Autodesk Inventor part; units mm, degrees
ref_plane "YZ Plane" through (0, 0, 0) normal (1, 0, 0) x (0, 1, 0)
ref_plane "XZ Plane" through (0, 0, 0) normal (0, 1, 0) x (-1, 0, 0)
ref_plane "XY Plane" through (0, 0, 0) normal (0, 0, 1) x (1, 0, 0)
sketch "Sketch1" plane through (0, 0, 0) normal (0, 0, 1) x (1, 0, 0)
  line L0 (-2.54, -8.19) -> (2.54, -8.19)
  line L1 (2.54, -8.19) -> (2.54, 8.19)
  line L2 (-2.54, 8.19) -> (-2.54, -8.19)
  line L3 (-2.54, -8.19) -> (2.54, 8.19) construction
  line L4 (2.54, -8.19) -> (-2.54, 8.19) construction
  circle A0 centre (0, 16.6545) radius 2.5 construction
  circle A1 centre (0, 16.6545) radius 5
  arc A2 (6.8029, 15.0051) -> (-6.8044, 15.0114) centre (0, 16.6545) ccw
  line L5 (-2.54, 8.19) -> (-2.54, 10.2591)
  line L6 (2.54, 8.19) -> (2.54, 10.2869)
  line L7 (0, 0) -> (0, 10.7842) construction
  line L8 (-2.54, 10.2591) -> (-3.9944, 10.2511)
  line L9 (2.54, 10.2869) -> (3.9944, 10.2948)
  line L10 (-3.9944, 10.2511) -> (-4.1214, 3.9003)
  line L11 (3.9944, 10.2948) -> (4.1214, 3.9454)
  line L12 (-4.1214, 3.9003) -> (-6.8044, 15.0114)
  line L13 (4.1214, 3.9454) -> (6.8029, 15.0051)
  line L14 (0, 0) -> (0, 22.9511) construction
  point P0 (-3.2672, 10.2551)
  dimension "d2" = 5
  dimension "d3" = 10
  dimension "d4" = 14
  dimension "d8" = 1.5815
  dimension "d9" = 1.5815
  dimension "d10" = 6.35
  dimension "d11" = 6.35
  dimension "d18" = 1.4545
  dimension "d19" = 1.4545
  dimension "d31" = 2.54
  dimension "d32" = 2.54
  dimension "d33" = 0
extrude "Plate1" add sketch "Sketch1" along normal blind 1.5748
sketch "Sketch2" plane through (0, 0, 0) normal (0, 0, -1) x (-1, 0, 0)
  circle A0 centre (0, 16.6545) radius 5
  line L0 (-3.9944, 10.2948) -> (-4.1214, 3.9454)
  line L1 (-2.54, 10.2869) -> (-3.9944, 10.2948)
  line L2 (-2.54, -8.19) -> (-2.54, 10.2869)
  line L3 (2.54, -8.19) -> (-2.54, -8.19)
  line L4 (2.54, 10.2591) -> (2.54, -8.19)
  line L5 (3.9944, 10.2511) -> (2.54, 10.2591)
  line L6 (4.1214, 3.9003) -> (3.9944, 10.2511)
  line L7 (6.8044, 15.0114) -> (4.1214, 3.9003)
  arc A1 (6.8044, 15.0114) -> (-6.8029, 15.0051) centre (0, 16.6545) ccw
  line L8 (-4.1214, 3.9454) -> (-6.8029, 15.0051)
  line L9 (-1.5875, -17.19) -> (1.5875, -17.19)
  line L10 (1.5875, -17.19) -> (1.5875, 0.81)
  line L11 (1.5875, 0.81) -> (-1.5875, 0.81)
  line L12 (-1.5875, 0.81) -> (-1.5875, -17.19)
  line L13 (-1.5875, -17.19) -> (1.5875, 0.81) construction
  line L14 (1.5875, -17.19) -> (-1.5875, 0.81) construction
  point P0 (0, 0)
  point P1 (0, -8.19)
  dimension "d14" = 3.175
extrude "Extrusion1" cut sketch "Sketch2" against normal blind 25.4 contours L12 L11 L10 L3 | L3 L10 L9 L12
sketch "Sketch3" plane through (0, 0, 1.5748) normal (0, 0, 1) x (1, 0, 0)
  circle A0 centre (-37.757, 0) radius 3
  line L0 (-39.3445, -2.5456) -> (-36.1695, -2.5456)
  line L1 (-36.1695, -2.5456) -> (-36.1695, 2.5456)
  line L2 (-36.1695, 2.5456) -> (-39.3445, 2.5456)
  line L3 (-39.3445, 2.5456) -> (-39.3445, -2.5456)
  line L4 (-39.3445, -2.5456) -> (-36.1695, 2.5456) construction
  line L5 (-36.1695, -2.5456) -> (-39.3445, 2.5456) construction
  circle A1 centre (-37.757, 0) radius 4
  point P0 (0, 0)
  point P1 (-37.757, 3)
  point P2 (-37.757, 4)
  dimension "d35" = 8
  dimension "d28" = 6
  dimension "d29" = 3.175
  dimension "d30" = 5.0911
  dimension "d34" = 0.4545
  dimension "d36" = 1.4545
fillet "Fillet4" radius 0.381 6 edges at (-4.1214, 3.9003, 0.7874) (4.1214, 3.9454, 0.7874) (-2.54, -8.19, 0.7874) (-1.5875, -8.19, 0.7874) (1.5875, -8.19, 0.7874) (2.54, -8.19, 0.7874)
sketch "Sketch4" plane through (0, 0, 1.5748) normal (0, 0, 1) x (1, 0, 0)
  arc A0 (2.159, -8.19) -> (2.54, -7.809) centre (2.159, -7.809) ccw
  line L0 (2.54, 10.2869) -> (2.54, -7.809)
  line L1 (3.9944, 10.2948) -> (2.54, 10.2869)
  line L2 (4.0627, 6.8835) -> (3.9944, 10.2948)
  arc A1 (4.0627, 6.8835) -> (4.8139, 6.8013) centre (4.4436, 6.8911) ccw
  line L3 (6.8029, 15.0051) -> (4.8139, 6.8013)
  arc A2 (6.8029, 15.0051) -> (-6.8044, 15.0114) centre (0, 16.6545) ccw
  line L4 (-4.8137, 6.7674) -> (-6.8044, 15.0114)
  arc A3 (-4.8137, 6.7674) -> (-4.0625, 6.8492) centre (-4.4434, 6.8568) ccw
  line L5 (-3.9944, 10.2511) -> (-4.0625, 6.8492)
  line L6 (-2.54, 10.2591) -> (-3.9944, 10.2511)
  line L7 (-2.54, -7.809) -> (-2.54, 10.2591)
  arc A4 (-2.54, -7.809) -> (-2.159, -8.19) centre (-2.159, -7.809) ccw
  line L8 (-1.9685, -8.19) -> (-2.159, -8.19)
  arc A5 (-1.9685, -8.19) -> (-1.5875, -7.809) centre (-1.9685, -7.809) ccw
  line L9 (-1.5875, -7.809) -> (-1.5875, 0.81)
  line L10 (-1.5875, 0.81) -> (1.5875, 0.81)
  line L11 (1.5875, 0.81) -> (1.5875, -7.809)
  arc A6 (1.5875, -7.809) -> (1.9685, -8.19) centre (1.9685, -7.809) ccw
  line L12 (2.159, -8.19) -> (1.9685, -8.19)
  circle A7 centre (0, 16.6545) radius 5
  point P0 (0, 0)
extrude "Extrusion2" add sketch "Sketch4" against normal up to surface (1.5748 mm away) contours A7
sketch "Sketch5" plane through (0, 0, 1.5748) normal (0, 0, 1) x (1, 0, 0)
  arc A0 (2.159, -8.19) -> (2.54, -7.809) centre (2.159, -7.809) ccw
  line L0 (2.54, 10.2869) -> (2.54, -7.809)
  line L1 (3.9944, 10.2948) -> (2.54, 10.2869)
  line L2 (4.0627, 6.8835) -> (3.9944, 10.2948)
  arc A1 (4.0627, 6.8835) -> (4.8139, 6.8013) centre (4.4436, 6.8911) ccw
  line L3 (6.8029, 15.0051) -> (4.8139, 6.8013)
  arc A2 (6.8029, 15.0051) -> (-6.8044, 15.0114) centre (0, 16.6545) ccw
  line L4 (-4.8137, 6.7674) -> (-6.8044, 15.0114)
  arc A3 (-4.8137, 6.7674) -> (-4.0625, 6.8492) centre (-4.4434, 6.8568) ccw
  line L5 (-3.9944, 10.2511) -> (-4.0625, 6.8492)
  line L6 (-2.54, 10.2591) -> (-3.9944, 10.2511)
  line L7 (-2.54, -7.809) -> (-2.54, 10.2591)
  arc A4 (-2.54, -7.809) -> (-2.159, -8.19) centre (-2.159, -7.809) ccw
  line L8 (-1.9685, -8.19) -> (-2.159, -8.19)
  arc A5 (-1.9685, -8.19) -> (-1.5875, -7.809) centre (-1.9685, -7.809) ccw
  line L9 (-1.5875, -7.809) -> (-1.5875, 0.81)
  line L10 (-1.5875, 0.81) -> (1.5875, 0.81)
  line L11 (1.5875, 0.81) -> (1.5875, -7.809)
  arc A6 (1.5875, -7.809) -> (1.9685, -8.19) centre (1.9685, -7.809) ccw
  line L12 (2.159, -8.19) -> (1.9685, -8.19)
  arc A7 (1.5644, 14.7045) -> (-1.5644, 14.7045) centre (0, 16.6545) ccw
  line L13 (1.5644, 14.7045) -> (-1.5644, 14.7045)
  point P0 (0, 0)
  point P1 (0, 19.1545)
  dimension "d40" = 5
  dimension "d44" = 4.45
extrude "Extrusion3" cut sketch "Sketch5" against normal blind 25.4 contours L13 A7
sketch "Sketch6" plane through (0, 0, 1.5748) normal (0, 0, 1) x (1, 0, 0)
  circle A0 centre (-0.0066, 22.9731) radius 10.9474
  line L0 (3.9944, 10.2948) -> (2.54, 10.2869)
  point P0 (0, 0)
  dimension "d45" = 21.8948
  dimension "d46" = 12.7
extrude "Extrusion4" add sketch "Sketch6" against normal up to surface (1.5748 mm away)
fillet "Fillet5" radius 3.175 2 edges at (-6.6204, 14.2495, 0.7874) (6.6225, 14.2611, 0.7874)
chamfer "Chamfer3" distance 3.175 angle 2 1 edges at (-2.54, 10.2591, 0.7874) measured on face at (-2.54, 4.2364, 0.5249)
chamfer "Chamfer4" distance 3.175 angle 2 1 edges at (2.54, 10.2869, 0.7874) measured on face at (2.54, -1.7771, 1.0499)
sketch "Sketch7" plane through (0, 0, 1.5748) normal (0, 0, 1) x (1, 0, 0)
  line L0 (-4.8137, 6.7674) -> (-6.3734, 13.2264)
  arc A0 (-4.8137, 6.7674) -> (-4.0625, 6.8492) centre (-4.4434, 6.8568) ccw
  line L1 (-3.9944, 10.2511) -> (-4.0625, 6.8492)
  line L2 (-2.6509, 10.2585) -> (-3.9944, 10.2511)
  line L3 (-2.54, 7.0841) -> (-2.6509, 10.2585)
  line L4 (-2.54, -7.809) -> (-2.54, 7.0841)
  arc A1 (-2.54, -7.809) -> (-2.159, -8.19) centre (-2.159, -7.809) ccw
  line L5 (-1.9685, -8.19) -> (-2.159, -8.19)
  arc A2 (-1.9685, -8.19) -> (-1.5875, -7.809) centre (-1.9685, -7.809) ccw
  line L6 (-1.5875, -7.809) -> (-1.5875, 0.81)
  line L7 (-1.5875, 0.81) -> (1.5875, 0.81)
  line L8 (1.5875, 0.81) -> (1.5875, -7.809)
  arc A3 (1.5875, -7.809) -> (1.9685, -8.19) centre (1.9685, -7.809) ccw
  line L9 (2.159, -8.19) -> (1.9685, -8.19)
  arc A4 (2.159, -8.19) -> (2.54, -7.809) centre (2.159, -7.809) ccw
  line L10 (2.54, 7.1119) -> (2.54, -7.809)
  line L11 (2.6509, 10.2875) -> (2.54, 7.1119)
  line L12 (3.9944, 10.2948) -> (2.6509, 10.2875)
  line L13 (4.0627, 6.8835) -> (3.9944, 10.2948)
  arc A5 (4.0627, 6.8835) -> (4.8139, 6.8013) centre (4.4436, 6.8911) ccw
  line L14 (6.3756, 13.2425) -> (4.8139, 6.8013)
  arc A6 (7.3326, 14.8503) -> (6.3756, 13.2425) centre (9.4612, 12.4944) ccw
  arc A7 (7.3326, 14.8503) -> (-7.3345, 14.84) centre (-0.0066, 22.9731) ccw
  arc A8 (-6.3734, 13.2264) -> (-7.3345, 14.84) centre (-9.4597, 12.4812) ccw
  circle A9 centre (-0.0066, 22.9731) radius 8
  point P0 (0, 0)
  point P1 (-0.0066, 14.9731)
  point P2 (-0.0066, 30.9731)
  point P3 (-8.0066, 22.9731)
  point P4 (7.9934, 22.9731)
  dimension "d56" = 16
hole "Hole1" at (-0.0066, 14.9731, 1.5748) at (-0.0066, 30.9731, 1.5748) at (-8.0066, 22.9731, 1.5748) at (7.9934, 22.9731, 1.5748) direction (0, 0, -1) diameter 2 end through all
sketch "Sketch8" plane through (0, 0, 1.5748) normal (0, 0, 1) x (1, 0, 0)
  circle A0 centre (-8.0066, 22.9731) radius 1
  circle A1 centre (-0.0066, 14.9731) radius 1
  circle A2 centre (-0.0066, 30.9731) radius 1
  circle A3 centre (7.9934, 22.9731) radius 1
  line L0 (-4.8137, 6.7674) -> (-6.3734, 13.2264)
  arc A4 (-4.8137, 6.7674) -> (-4.0625, 6.8492) centre (-4.4434, 6.8568) ccw
  line L1 (-3.9944, 10.2511) -> (-4.0625, 6.8492)
  line L2 (-2.6509, 10.2585) -> (-3.9944, 10.2511)
  line L3 (-2.54, 7.0841) -> (-2.6509, 10.2585)
  line L4 (-2.54, -7.809) -> (-2.54, 7.0841)
  arc A5 (-2.54, -7.809) -> (-2.159, -8.19) centre (-2.159, -7.809) ccw
  line L5 (-1.9685, -8.19) -> (-2.159, -8.19)
  arc A6 (-1.9685, -8.19) -> (-1.5875, -7.809) centre (-1.9685, -7.809) ccw
  line L6 (-1.5875, -7.809) -> (-1.5875, 0.81)
  line L7 (-1.5875, 0.81) -> (1.5875, 0.81)
  line L8 (1.5875, 0.81) -> (1.5875, -7.809)
  arc A7 (1.5875, -7.809) -> (1.9685, -8.19) centre (1.9685, -7.809) ccw
  line L9 (2.159, -8.19) -> (1.9685, -8.19)
  arc A8 (2.159, -8.19) -> (2.54, -7.809) centre (2.159, -7.809) ccw
  line L10 (2.54, 7.1119) -> (2.54, -7.809)
  line L11 (2.6509, 10.2875) -> (2.54, 7.1119)
  line L12 (3.9944, 10.2948) -> (2.6509, 10.2875)
  line L13 (4.0627, 6.8835) -> (3.9944, 10.2948)
  arc A9 (4.0627, 6.8835) -> (4.8139, 6.8013) centre (4.4436, 6.8911) ccw
  line L14 (6.3756, 13.2425) -> (4.8139, 6.8013)
  arc A10 (7.3326, 14.8503) -> (6.3756, 13.2425) centre (9.4612, 12.4944) ccw
  arc A11 (7.3326, 14.8503) -> (-7.3345, 14.84) centre (-0.0066, 22.9731) ccw
  arc A12 (-6.3734, 13.2264) -> (-7.3345, 14.84) centre (-9.4597, 12.4812) ccw
  line L15 (-15.0886, 10.1904) -> (17.7412, 10.3701)
  line L16 (17.7412, 10.3701) -> (17.8596, -11.273)
  line L17 (17.8596, -11.273) -> (-14.9701, -11.4526)
  line L18 (-14.9701, -11.4526) -> (-15.0886, 10.1904)
  point P0 (0, 0)
extrude "Extrusion5" cut sketch "Sketch8" against normal blind 25.4 contours A4 L1 L2 L3 L4 A5 L5 A6 L6 L7 L8 A7 L9 A8 L10 L11 L12 L13 A9 L14 L15 L16 L17 L18 L0 | L0 L15 L1 A4 | L15 L11 L10 A8 L9 A7 L8 L7 L6 A6 L5 A5 L4 L3 | L15 L14 A9 L13
fillet "Fillet6" radius 3.175 2 edges at (-5.6528, 10.2421, 0.7874) (5.6631, 10.304, 0.7874)
equation "\"d18\" = d36"
equation "\"d19\" = d36"
equation "\"d62\" = Thickness"
equation "\"BendRadius\" = Thickness"
equation "\"BendReliefWidth\" = Thickness"
equation "\"BendReliefDepth\" = 0.5 * Thickness"
equation "\"CornerReliefSize\" = 4 * Thickness"
equation "\"MinimumRemnant\" = 2 * Thickness"
equation "\"TransitionRadius\" = BendRadius"
equation "\"JacobiRadiusSize\" = BendRadius"
equation "\"GapSize\" = Thickness"
equation "\"d12\" = BendRadius"
properties part number "8mm OD 6mm ID Rod End125DynamixelSpacer"
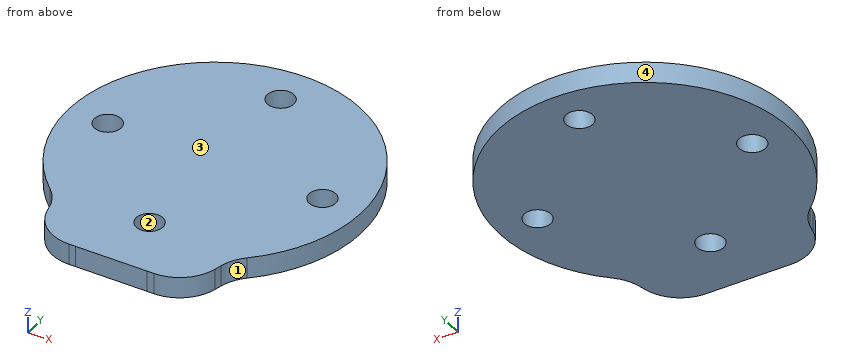
Here's how the part is built. I have some questions about the finished solid (model axes, mm). Face numbers are marked on the shaded views. Coordinates: 2 decimals unless noted, no trailing zeros. Loops run counter-clockwise (first coordinate to the right, second up) from the corner with the lowest first, then second, coordinate; pieces in that order, holes last.
1. Imagine slicing it at D-D, the plane x = -9.5. Please give me the cut outline in (y, z).
2. I need wall thicknesses on L1, parallel to X at y = 23.5, z = 1.1; L2, parallel to X at y = 22.5, z = 0.35; L3, parallel to Y at x = -8.25, z = 1.05. Which ranges of each line are inside material? Lowest first, please.
3. If we mould it in two halves opening along X, with no side actions, what happens to the marked faces 1, 2, 3 and 4? For each: pulls with the +X half, pulls with the -X half, needs draft (parallel to the pull), parting line crosses it, or undercut.
4. Imagine slicing it at C-C, the plane y = 15.5. Please give me the cut outline in (x, z).
5. Imagine slicing it at A-A, the plane y = 31. Please give me the cut outline in (x, z).
6. Imagine slicing it at B-B, the plane y = 22.5. Please give me the cut outline in (x, z), and give its area (3 significant figures).
Taken from the geometry:
1. outline: (17.52, 0) - (28.42, 0) - (28.42, 1.57) - (17.52, 1.57) - close
2. L1: x = -10.94 to -8.86, -7.16 to 7.14, 8.84 to 10.93
2. L2: x = -10.94 to -8.89, -7.13 to 7.11, 8.87 to 10.93
2. L3: y = 15.77 to 22, 23.94 to 30.18
3. face 1: pulls with the +X half
3. face 2: undercut
3. face 3: needs draft
3. face 4: parting line crosses it
4. outline: (-8.01, 0) - (-0.86, 0) - (-0.86, 1.57) - (-8.01, 1.57) - close; (0.84, 0) - (7.99, 0) - (7.99, 1.57) - (0.84, 1.57) - close
5. outline: (-7.45, 0) - (-1.01, 0) - (-1.01, 1.57) - (-7.45, 1.57) - close; (0.99, 0) - (7.44, 0) - (7.44, 1.57) - (0.99, 1.57) - close
6. outline: (-10.94, 0) - (-8.89, 0) - (-8.89, 1.57) - (-10.94, 1.57) - close; (-7.13, 0) - (7.11, 0) - (7.11, 1.57) - (-7.13, 1.57) - close; (8.87, 0) - (10.93, 0) - (10.93, 1.57) - (8.87, 1.57) - close
6. area: 28.9 mm2
